For this review, take the finished solid that the model builds, in its own axes (mm). Give positions to 0.01 mm unless a question says otherwise; leave off trailing zeros. Order: outer loops, then holes, each group sorted by start corner. A loop starts at its lowest first (then second) coordinate and runs counter-clockwise, first axis right, second up. Notation, with made-up numbers: (4, 77) -> (23, 77) arc R15 ccw to (23, 102) -> close; hole circle Ø5 at (26, 46.5). An arc over 180 degrees is marked (long way). Return JSON: item names as keys, results as strings. Group by question number.
1) Insertion check: P1, Ø8, axis at x = 20, z = 6.5, coming from the -Y side; P2, Ø12, axis at x = 3.5, y = 248, coming from the +Z side; P3, Ø12, axis at y = 687, z = 3.5, coming from the +X side; P4, Ø12, axis at x = 7, z = 8, coming from the -Y side. Each pin has a flat end and moves straight along its axis. Give the tip position at first contact, or say it passes through.
2) To check wall thickness, follow line 1 along Y through (x, z) = (0, -1.75); line 2 along X through (y, z) = (0, 0.25); line 3 along Y through (x, z) = (46.5, -2.5). State the ranges of each line that lie inside material, in increasing order.
3) Add section B-B (x = 22). Give the boundary of the cut face in (y, z), then the cut area to 3 significant figures.
4) Add section A-A (y = 427). Give the boundary of the cut face in (x, z).
5) Add section C-C (y = 798). Give the boundary of the cut face in (x, z).
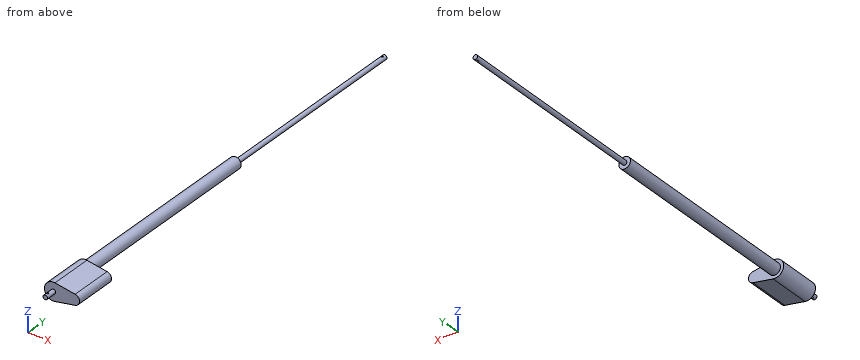
from build123d import *

# Parameters (mm, degrees)
CUT_EXTRUDE2_DEPTH      = 1034.387149136
CUT_EXTRUDE2_DEPTH_BACK = 1034.387149136
SKETCH8_R               = 2
BOSS_EXTRUDE4_DEPTH     = 98


with BuildPart() as part:
    # Sketch7 → Revolve2 (revolve)
    with BuildSketch(Plane(origin=(0, 0, 0), x_dir=(0, 0, -1), z_dir=(1, 0, 0))):
        Polygon((-20, 17), (-20, 115), (-13, 115), (-13, 575), (-5, 575), (-5, 1033), (0, 1033), (0, -8), (-5, -8), (-5, 17), align=None)
    revolve(axis=Axis((0, 1033, 0), (0, -1, 0)))

    # Sketch8 → Cut-Extrude2 (cut, two sides: drawn at the far end of the back side and taken through both)
    with BuildSketch(Plane.XY.offset(-CUT_EXTRUDE2_DEPTH_BACK)):
        with Locations((0, 1025)):
            Circle(SKETCH8_R)
        Circle(SKETCH8_R)
    extrude(amount=CUT_EXTRUDE2_DEPTH + CUT_EXTRUDE2_DEPTH_BACK, mode=Mode.SUBTRACT)

    # Sketch10 → Boss-Extrude4 (add)
    with BuildSketch(Plane(origin=(0, 115, 0), x_dir=(1, 0, 0), z_dir=(0, 1, 0))):
        with BuildLine():
            Line((3.491027189, 19.692961412), (48.629242089, 11.691181882))
            ThreePointArc((48.629242089, 11.691181882), (58.430175518, 0), (48.629242089, -11.691181882))
            Line((48.629242089, -11.691181882), (3.491027189, -19.692961412))
            ThreePointArc((3.491027189, -19.692961412), (-20, 0), (3.491027189, 19.692961412))
        make_face()
    extrude(amount=-BOSS_EXTRUDE4_DEPTH)


solid = part.part
Evaluation:
{
 "1": {"P1": "y = 17", "P2": "z = 13", "P3": "x = 5", "P4": "y = -8"},
 "2": {"line 1": "-8 to -2, 2 to 1023, 1027 to 1033", "line 2": "-4.99 to -2, 2 to 4.99", "line 3": "17 to 115"},
 "3": {"outline": "(17, -16.41) -> (115, -16.41) -> (115, 16.41) -> (17, 16.41) -> close", "area": "3,220 mm^2"},
 "4": {"outline": "circle Ø26 at (0, 0)"},
 "5": {"outline": "circle Ø10 at (0, 0)"}
}
